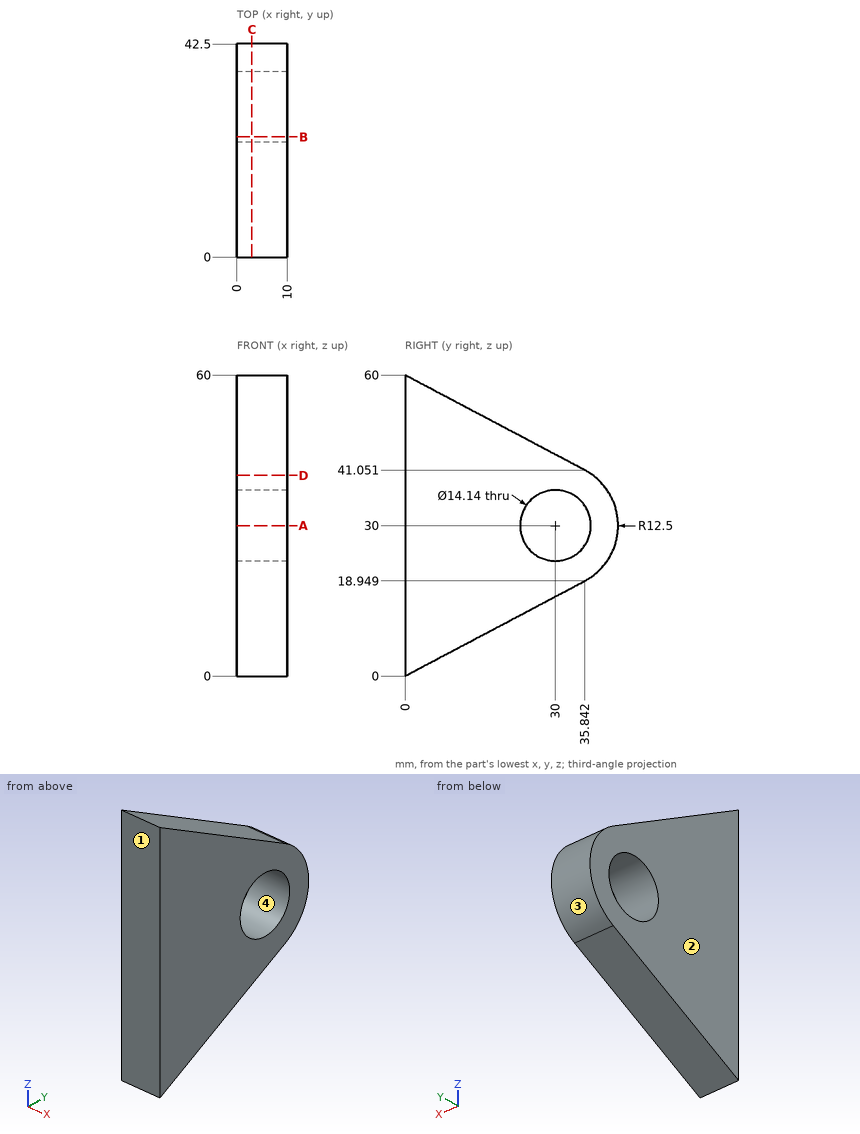
Part print with two shaded views. Sizes in mm from the minimum x, y, z corner. Round coordinates to 2 decimals unless told otherwise and drop trailing zeros. Order: outer loops, then holes, each group sorted by start corner. A loop starts at its lowest first (then second) coordinate and runs counter-clockwise, first axis right, second up. Notation, with made-up numbers: (-27.5, 85) - (4.5, 85) arc R17 ccw to (4.5, 96) - close; hole circle Ø3 at (20, 19.25). An arc over 180 degrees is marked (long way). Answer as CSV lines item,"result". Start each with the question number.
1. Saw through at A-A, the plane z = 30. Write the cut outline in (x, y).
2. Saw through at D-D, the plane z = 40. Write the cut outline in (x, y).
3. Pull direction Y, two halves, no side cores. Call the marked faces 1, 2, 3 and 4: +Y half, -Y half, draft (parallel to the pull), parting line (faces both ways), or undercut.
4. Saw through at C-C, the plane x = 3. Write the cut outline in (y, z).
5. Pin check, flat tips, straight feed: pin 1 (2 mm diameter, centred on x = 1, z = 53.5, fed in from +Y) (1 decimal); pin 2 (1.5 mm diameter, centred on x = 3.5, y = 21, fed in from -Z) (1 decimal); pin 3 (5 mm diameter, centred on x = 2, y = 37, fed in from +Z). Stop position of each tip, or through.
6. Drill centre lines: L1, parallel to Y at x = 2.25, z = 31.5; L2, parallel to Z at x = 8, y = 34.5; L3, parallel to Z at x = 8.25, y = 30. Where is each one in solid material? Low to high. Write a range as [from, to].
7. Saw through at B-B, the plane y = 24. Write the cut outline in (x, z).
Model answer:
1,outline,"(0, 0) - (10, 0) - (10, 22.93) - (0, 22.93) - close; (0, 37.07) - (10, 37.07) - (10, 42.5) - (0, 42.5) - close"
2,outline,"(0, 0) - (10, 0) - (10, 37.5) - (0, 37.5) - close"
3,face 1,"-Y half"
3,face 2,"draft"
3,face 3,"+Y half"
3,face 4,"undercut"
4,outline,"(0, 0) - (35.84, 18.95) arc R12.5 ccw to (35.84, 41.05) - (0, 60) - close; hole circle Ø14.14 at (30, 30)"
5,pin 1,"stops at y = 14.2"
5,pin 2,"stops at z = 10.7"
5,pin 3,"stops at z = 41.76"
6,L1,"y = [0, 23.09], [36.91, 42.41]"
6,L2,"z = [18.24, 24.55], [35.45, 41.76]"
6,L3,"z = [15.86, 22.93], [37.07, 44.14]"
7,outline,"(0, 12.69) - (10, 12.69) - (10, 26.26) - (0, 26.26) - close; (0, 33.74) - (10, 33.74) - (10, 47.31) - (0, 47.31) - close"
